```python
from build123d import *

# Parameters (mm, degrees)
SKETCH1_W                = 60.5
SKETCH1_H                = 53.5
SKETCH1_R                = 1.65
BOSS_EXTRUDE1_DEPTH      = 1.56
SKETCH2_W                = 59.3
SKETCH2_H                = 41.3
BOSS_EXTRUDE2_DEPTH      = 5
SKETCH4_W                = 41.5
SKETCH4_H                = 5
CUT_EXTRUDE1_DEPTH       = 1
BOSS_EXTRUDE3_DEPTH      = 6.05
BOSS_EXTRUDE3_DEPTH_BACK = 6.05
SKETCH5_W                = 15.8
SKETCH5_H                = 2.5
SKETCH5_W_2              = 20.8
SKETCH5_W_3              = 25.9
BOSS_EXTRUDE4_DEPTH      = 8.4
SKETCH6_W                = 3.5
SKETCH6_H                = 7
BOSS_EXTRUDE5_DEPTH      = 4
SKETCH7_W                = 57.2
SKETCH7_H                = 8
CUT_EXTRUDE2_DEPTH       = 1
SKETCH8_W                = 57.2
SKETCH8_H                = 31.25
CUT_EXTRUDE3_DEPTH       = 0.05
SKETCH9_W                = 5.6
SKETCH9_H                = 8
BOSS_EXTRUDE6_DEPTH      = 3
CUT_EXTRUDE4_DEPTH       = 5.6


with BuildPart() as part:
    # Sketch1 → Boss-Extrude1 (new body)
    with BuildSketch(Plane(origin=(0, 0, 0), x_dir=(1, 0, 0), z_dir=(0, 1, 0))):
        with Locations((-0.970473773, 6.36428867)):
            Rectangle(SKETCH1_W, SKETCH1_H)
        with Locations((-27.970473773, -16.88571133)):
            Circle(SKETCH1_R, mode=Mode.SUBTRACT)
        with Locations((-27.970473773, 29.61428867)):
            Circle(SKETCH1_R, mode=Mode.SUBTRACT)
        with Locations((26.029526227, 29.61428867)):
            Circle(SKETCH1_R, mode=Mode.SUBTRACT)
        with Locations((26.029526227, -16.88571133)):
            Circle(SKETCH1_R, mode=Mode.SUBTRACT)
    extrude(amount=BOSS_EXTRUDE1_DEPTH)

    # Sketch2 → Boss-Extrude2 (add)
    with BuildSketch(Plane(origin=(0, 1.56, 0), x_dir=(1, 0, 0), z_dir=(0, 1, 0))):
        with Locations((-0.970473773, 6.96428867)):
            Rectangle(SKETCH2_W, SKETCH2_H)
    extrude(amount=BOSS_EXTRUDE2_DEPTH)

    # Sketch4 → Cut-Extrude1 (cut)
    with BuildSketch(Plane.XY.offset(13.68571133)):
        with Locations((-0.970473773, 4.06)):
            Rectangle(SKETCH4_W, SKETCH4_H)
    extrude(amount=-CUT_EXTRUDE1_DEPTH, mode=Mode.SUBTRACT)

    # Sketch3 → Boss-Extrude3 (add, two sides)
    with BuildSketch(Plane(origin=(0, 0, 0), x_dir=(0, 0, -1), z_dir=(1, 0, 0))) as boss_extrude3_sk:
        with BuildLine():
            Line((-11.68571133, 5.41), (-11.68571133, 5.56))
            ThreePointArc((-11.68571133, 5.56), (-14.583986679, 4.399736831), (-15.880946723, 1.56))
            Line((-15.880946723, 1.56), (-15.730770044, 1.56))
            ThreePointArc((-15.730770044, 1.56), (-14.4778879, 4.293641082), (-11.68571133, 5.41))
        make_face()
    extrude(amount=BOSS_EXTRUDE3_DEPTH)
    extrude(boss_extrude3_sk.sketch, amount=-BOSS_EXTRUDE3_DEPTH_BACK)

    # Sketch5 → Boss-Extrude4 (add)
    with BuildSketch(Plane(origin=(0, 0, 0), x_dir=(-1, 0, 0), z_dir=(0, -1, 0))):
        with Locations((17.120473773, -17.73571133)):
            Rectangle(SKETCH5_W, SKETCH5_H)
        with Locations((-3.479526227, -17.73571133)):
            Rectangle(SKETCH5_W_2, SKETCH5_H)
        with Locations((14.620473773, 30.46428867)):
            Rectangle(SKETCH5_W_2, SKETCH5_H)
        with Locations((-9.729526227, 30.46428867)):
            Rectangle(SKETCH5_W_3, SKETCH5_H)
    extrude(amount=BOSS_EXTRUDE4_DEPTH)

    # Sketch6 → Boss-Extrude5 (add)
    with BuildSketch(Plane.XZ):
        with Locations((-29.270473773, 0.78571133)):
            Rectangle(SKETCH6_W, SKETCH6_H)
        with Locations((-29.270473773, -20.61428867)):
            Rectangle(SKETCH6_W, SKETCH6_H)
        with Locations((27.329526227, 0.78571133)):
            Rectangle(SKETCH6_W, SKETCH6_H)
        with Locations((27.329526227, -20.61428867)):
            Rectangle(SKETCH6_W, SKETCH6_H)
    extrude(amount=BOSS_EXTRUDE5_DEPTH)

    # Sketch7 → Cut-Extrude2 (cut)
    with BuildSketch(Plane(origin=(0, 6.56, 0), x_dir=(1, 0, 0), z_dir=(0, 1, 0))):
        with Locations((-0.970473773, -8.68571133)):
            Rectangle(SKETCH7_W, SKETCH7_H)
    extrude(amount=-CUT_EXTRUDE2_DEPTH, mode=Mode.SUBTRACT)

    # Sketch8 → Cut-Extrude3 (cut)
    with BuildSketch(Plane(origin=(0, 6.56, 0), x_dir=(1, 0, 0), z_dir=(0, 1, 0))):
        with Locations((-0.970473773, 10.93928867)):
            Rectangle(SKETCH8_W, SKETCH8_H)
    extrude(amount=-CUT_EXTRUDE3_DEPTH, mode=Mode.SUBTRACT)

    # Sketch9 → Boss-Extrude6 (add)
    with BuildSketch(Plane(origin=(0, 0, 0), x_dir=(-1, 0, 0), z_dir=(0, -1, 0))):
        with Locations((-26.729526227, 10.11428867)):
            Rectangle(SKETCH9_W, SKETCH9_H)
    extrude(amount=BOSS_EXTRUDE6_DEPTH)

    # Sketch10 → Cut-Extrude4 (cut)
    with BuildSketch(Plane(origin=(29.529526227, 0, 0), x_dir=(0, 0, -1), z_dir=(1, 0, 0))):
        with BuildLine():
            Line((7.436374303, 0), (6.278331815, -1.852433806))
            ThreePointArc((6.278331815, -1.852433806), (6.258287662, -2.613541851), (6.91428867, -3))
            Line((6.91428867, -3), (6.11428867, -3))
            Line((6.11428867, -3), (6.11428867, 0))
            Line((6.11428867, 0), (7.436374303, 0))
        make_face()
        with BuildLine():
            Line((12.792203037, 0), (13.950245525, -1.852433806))
            ThreePointArc((13.950245525, -1.852433806), (13.970289678, -2.613541851), (13.31428867, -3))
            Line((13.31428867, -3), (14.11428867, -3))
            Line((14.11428867, -3), (14.11428867, 0))
            Line((14.11428867, 0), (12.792203037, 0))
        make_face()
    extrude(amount=-CUT_EXTRUDE4_DEPTH, mode=Mode.SUBTRACT)


solid = part.part
```
Input: part model. Units: mm. Frame: model coordinates. A direction names the side the tool comes from. Give positions to 0.01 mm unless a question says otherwise; leave off trailing zeros. Loops run counter-clockwise (first coordinate to the right, second up) from the corner with the lowest first, then second, coordinate; pieces in that order, holes last. Notation, with made-up numbers: M 89,68 L 133,68 A14 cw 133,93 Z; hole C -12.75,-11.5 d10. An arc over 180 degrees is marked long. Answer as CSV lines item,"result". Start each with the question number.
1. Section A-A on y = -6.5. Return loops of the section in (x, z).
2. Section B-B on x = 18.5. Return loops of the section in (y, z), plus the area to 3 significant figures.
3. Reachability of faces 4 (the face through (22.68, -4, -30)), 5 (the face through (-1, 5.56, 9)), 6 (the face through (10, -4, -31.714)), 7 (the face through (-17, -4, 16.486)), 8 (the face through (0.08, 3.9, 14.84)) from +Z, -Z, +X, -X, +Y, -Y: full face, straight path, thin tool, end or side. Return the list, or none.
4. Pin query (flat end, axial travel): P1, Ø1, axis at x = -17, z = 6.5, coming from the +Y side; P2, Ø5, axis at x = 20, y = 4.5, coming from the -Z side; P3, Ø5, axis at x = 2, y = 2, coming from the -Z side; P4, Ø1.5, axis at x = -10, z = -23, coming from the +Y side. Return the tip coordinate at first contact, or that it passes through.
5. Pull-direction query (X, two-part tool) for faces 1 (the face through (-0.08, 4.86, 14.01)), 2 (the face through (10, -4, -29.214)), 3 (the face through (-31.22, 1, -6)); classes: released by +X, released by -X, zero draft, split by the parting line, or undercut.
6. Line query: L1, parallel to X at y = 5.25, z = 13; L2, parallel to Z at x = -25, y = 5.75; L3, parallel to Z at x = -24.5, y = -2. Output: solid intervals per line, ascending.
7. Section D-D on x = 2. Return loops of the section in (y, z), plus the area to 3 significant figures.
8. Section C-C on z = -5. Return loops of the section in (x, y).
Computed values:
1,outline,"M -25.02,-31.71 L -4.22,-31.71 L -4.22,-29.21 L -25.02,-29.21 Z; M -25.02,16.49 L -9.22,16.49 L -9.22,18.99 L -25.02,18.99 Z; M -6.92,16.49 L 13.88,16.49 L 13.88,18.99 L -6.92,18.99 Z; M -3.22,-31.71 L 22.68,-31.71 L 22.68,-29.21 L -3.22,-29.21 Z"
2,outline,"M -8.4,-31.71 L 0,-31.71 L 0,-33.11 L 1.56,-33.11 L 1.56,-27.61 L 6.56,-27.61 L 6.56,-26.56 L 6.51,-26.56 L 6.51,4.69 L 5.56,4.69 L 5.56,12.69 L 1.56,12.69 L 1.56,20.39 L 0,20.39 L 0,-29.21 L -8.4,-29.21 Z"
2,area,"296 mm²"
3,face 4,"+Z, -Z, +X, -Y"
3,face 5,"+Y"
3,face 6,"-Z, +X, -X, -Y"
3,face 7,"+X, -X, -Y"
3,face 8,"none"
4,P1,"stops at y = 5.56"
4,P2,"stops at z = -27.61"
4,P3,"stops at z = -33.11"
4,P4,"stops at y = 6.51"
5,face 1,"undercut"
5,face 2,"zero draft"
5,face 3,"released by -X"
6,L1,"x = -30.62 to -21.72, -6.05 to 6.05, 19.78 to 28.68"
6,L2,"z = -27.61 to 4.69, 12.69 to 13.69"
6,L3,"z = -31.71 to -29.21, 16.49 to 18.99"
7,outline,"M -8.4,-31.71 L 0,-31.71 L 0,-33.11 L 1.56,-33.11 L 1.56,-27.61 L 6.56,-27.61 L 6.56,-26.56 L 6.51,-26.56 L 6.51,4.69 L 5.56,4.69 L 5.56,12.69 L 5.44,12.69 A4.2 ccw 1.56,15.88 L 1.56,20.39 L 0,20.39 L 0,18.99 L -8.4,18.99 L -8.4,16.49 L 0,16.49 L 0,-29.21 L -8.4,-29.21 Z; hole M 1.56,12.69 L 5.28,12.69 A4.05 ccw 1.56,15.73 Z"
7,area,"318 mm²"
8,outline,"M -31.22,0 L 29.28,0 L 29.28,1.56 L 28.68,1.56 L 28.68,6.56 L 27.63,6.56 L 27.63,6.51 L -29.57,6.51 L -29.57,6.56 L -30.62,6.56 L -30.62,1.56 L -31.22,1.56 Z"
